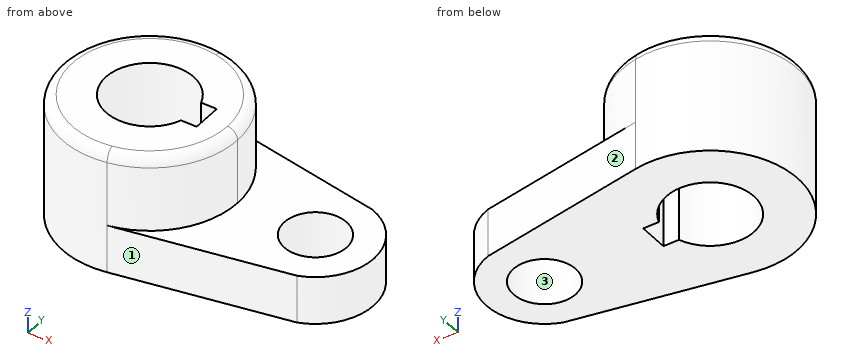
from build123d import *

# Parameters (mm, degrees)
F0_R     = 10.16
F1_DEPTH = 15.7734
F3_DEPTH = 24.4602
F5_DEPTH = 40.2346
F6_R     = 3.302


with BuildPart() as f1:
    # F0 (on Top) → F1 (new body)
    with BuildSketch(Plane.XY):
        with BuildLine():
            Line((60.155679, 18.019481), (5.154464, 28.106265))
            ThreePointArc((5.154464, 28.106265), (-28.575, -0.002611), (5.159601, -28.105322))
            Line((5.159601, -28.105322), (60.22005, -17.997273))
            ThreePointArc((60.22005, -17.997273), (73.02497, 0.034047), (60.155679, 18.019481))
        make_face()
        with Locations((53.975, 0)):
            Circle(F0_R, mode=Mode.SUBTRACT)
    extrude(amount=F1_DEPTH)

    # F2 (on face) → F3 (join)
    with BuildSketch(Plane.XY.offset(15.7734)):
        with BuildLine():
            ThreePointArc((5.159601, -28.105322), (21.954114, -18.29064), (28.575, 0))
            ThreePointArc((28.575, 0), (21.952442, 18.292646), (5.154464, 28.106265))
            ThreePointArc((5.154464, 28.106265), (-28.575, -0.002611), (5.159601, -28.105322))
        make_face()
    extrude(amount=F3_DEPTH)

    # F4 (on face) → F5 (cut, through all)
    with BuildSketch(Plane.XY.offset(40.2336)):
        with BuildLine():
            Line((18.5293, 4.826), (13.447765, 4.826))
            ThreePointArc((13.447765, 4.826), (-14.2875, 0), (13.447765, -4.826))
            Line((13.447765, -4.826), (18.5293, -4.826))
            Line((18.5293, -4.826), (18.5293, 4.826))
        make_face()
    extrude(amount=-F5_DEPTH, mode=Mode.SUBTRACT)

    # F6
    f6_edges = [f1.edges().sort_by_distance(p)[0] for p in [
        (-5.159601, 28.105322, 40.2336),
    ]]
    fillet(f6_edges, radius=F6_R)


solid = f1.part
Verification items for the finished model (mm, model axes). Face numbers are marked on the shaded views. Give positions to 0.01 mm unless a question says otherwise; leave off trailing zeros. Order: outer loops, then holes, each group sorted by start corner. A loop starts at its lowest first (then second) coordinate and runs counter-clockwise, first axis right, second up. Notation, with made-up numbers: (55.5, -13) -> (80.5, -13) arc R20 cw to (80.5, 8) -> close; hole circle Ø1 at (21.5, 81.5). An arc over 180 degrees is marked (long way). Answer as CSV lines item,"result".
Q1. Scan lines: probe 1 along X at (y, z) = (-6, 2.5); probe 2 along Y at (x, z) = (0, 21.5) (1 decimal); probe 3 along X at (y, z) = (0, 30.5) (1 decimal). Record each from-to range of solid material in increasing order.
Solutions:
probe 1,"x = -27.94 to -12.97, 12.97 to 45.78, 62.17 to 72.06"
probe 2,"y = -28.6 to -14.3, 14.3 to 28.6"
probe 3,"x = -28.6 to -14.3, 18.5 to 28.6"
Q2. Sectioned sample at B-B on x = 45. Record the cut outline in (y, z), plus the area to 3 significant figures.
Solutions:
outline,"(-20.79, 0) -> (-4.76, 0) -> (-4.76, 15.77) -> (-20.79, 15.77) -> close; (4.76, 0) -> (20.8, 0) -> (20.8, 15.77) -> (4.76, 15.77) -> close"
area,"506 mm²"
Q3. Sectioned sample at A-A on z = 4. Count the separate pieces of the cut face and the enclosed holes in it, plus the area to 3 significant figures.
Solutions:
separate pieces,"1"
enclosed holes,"2"
area,"3,440 mm²"
Q4. Depth check by flat-ended pin: pin 1 (6 mm diameter, centred on y = 17.5, z = 23, fed in from +X); pin 2 (2 mm diameter, centred on y = 20.5, z = 34, fed in from +X); pin 3 (2.5 mm diameter, centred on x = 16.5, z = 29, fed in from +Y); pin 4 (4 mm diameter, centred on x = 56, y = -21.5, fed in from +Z). Enter the tip coordinate at first touch or a pass-through.
Solutions:
pin 1,"stops at x = 24.62"
pin 2,"stops at x = 20.89"
pin 3,"stops at y = 24.17"
pin 4,"passes through"
Q5. Release check for a two-part mould opening along Y. For the marked faces 1, 2 and 3 record: +Y half, -Y half, draft (parallel to the pull), parting line (faces both ways), or undercut.
Solutions:
face 1,"-Y half"
face 2,"+Y half"
face 3,"undercut"
